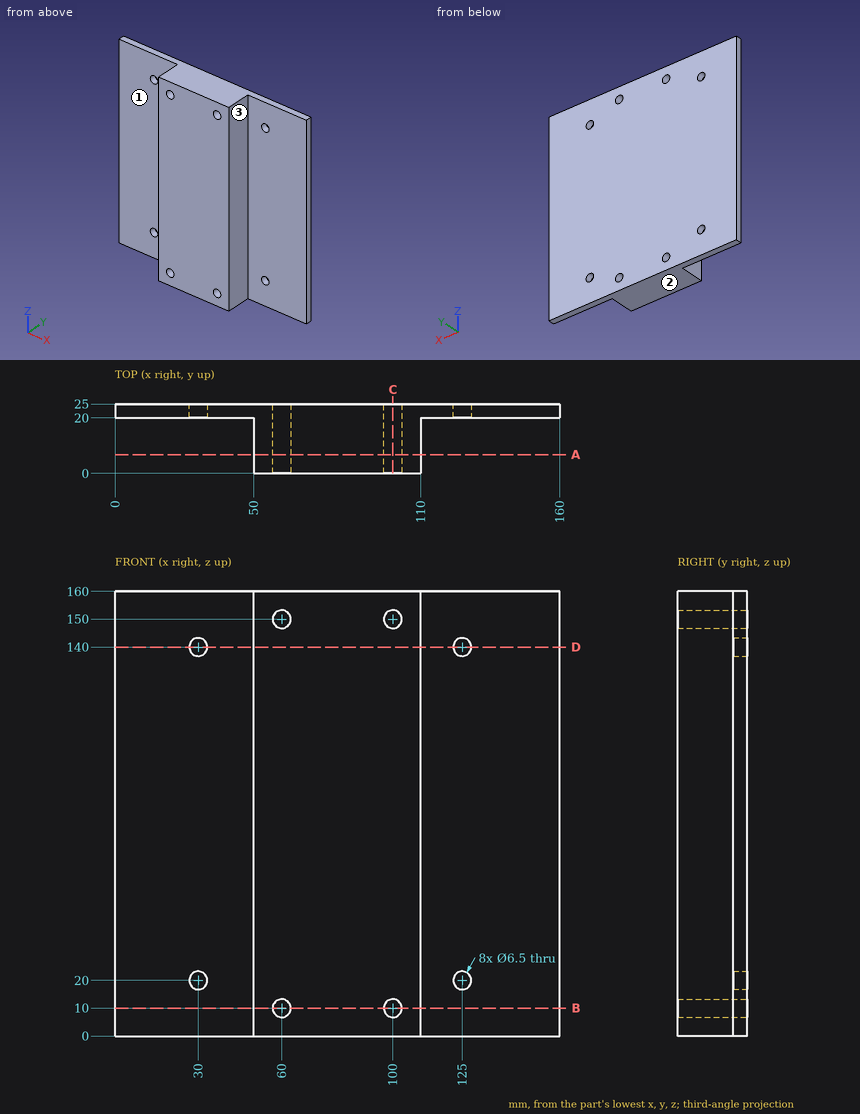
Job drawing, mm, ordinate dimensions from the low corner. One solid piece. A direction names the side the tool comes from. Coordinates: 2 decimals unless noted, no trailing zeros. Order: outer loops, then holes, each group sorted by start corner. A loop starts at its lowest first (then second) coordinate and runs counter-clockwise, first axis right, second up. Notation, with made-up numbers: (-38, 83.25) -> (-32, 83.25) arc R20 ccw to (-32, 118.25) -> close; hole circle Ø11 at (17, 36.5). An arc over 180 degrees is marked (long way). Put each result on its own line as item: value. Start each with the question number.
(1) Band-saw the part on A-A (y = 6.75). Give the cut face in (x, z), then the cut area to 3 significant figures.
(2) Band-saw the part on C-C (x = 100). Give the cut face in (y, z), then the cut area to 4 significant figures.
(3) Band-saw the part on B-B (z = 10). Give the cut face in (x, y), then the cut area to 4 significant figures.
(4) Probe line 1 along Z through (x, y) = (30, 22.05); line 2 along X through (y, z) = (5.5, 150); line 3 along Z through (x, y) = (100, 10). List the from-to ranges inside material, lowest first. Write a range as [from, to].
(5) Which spindle directions (+Z, -Z, +X, -X, +Y, -Y) get a long thin tool onto all of the face, cutting with end or side? Do the marked faces 1, 2 and 3. Say none if no direction does.
(6) Pin check, flat tips, straight feed: pin 1 Ø6 at (y, z) = (8.5, 112.5) entering from -X; pin 2 Ø15 at (x, z) = (135, 95) entering from -Y; pin 3 Ø4 at (x, z) = (30, 140) entering from +Y; pin 4 Ø4 at (y, z) = (15, 133) entering from +X. Stop position of each tip, or through.
(7) Band-saw the part on D-D (z = 140). Give the cut face in (x, y), then the cut area to 4 significant figures.
Determined:
1. outline: (50, 0) -> (110, 0) -> (110, 160) -> (50, 160) -> close; hole circle Ø6.5 at (60, 10); hole circle Ø6.5 at (60, 150); hole circle Ø6.5 at (100, 10); hole circle Ø6.5 at (100, 150)
1. area: 9,470 mm²
2. outline: (0, 0) -> (25, 0) -> (25, 6.75) -> (0, 6.75) -> close; (0, 13.25) -> (25, 13.25) -> (25, 146.75) -> (0, 146.75) -> close; (0, 153.25) -> (25, 153.25) -> (25, 160) -> (0, 160) -> close
2. area: 3,675 mm²
3. outline: (0, 20) -> (50, 20) -> (50, 0) -> (56.75, 0) -> (56.75, 25) -> (0, 25) -> close; (63.25, 0) -> (96.75, 0) -> (96.75, 25) -> (63.25, 25) -> close; (103.25, 0) -> (110, 0) -> (110, 20) -> (160, 20) -> (160, 25) -> (103.25, 25) -> close
3. area: 1,675 mm²
4. line 1: z = [0, 16.75], [23.25, 136.75], [143.25, 160]
4. line 2: x = [50, 56.75], [63.25, 96.75], [103.25, 110]
4. line 3: z = [0, 6.75], [13.25, 146.75], [153.25, 160]
5. face 1: +Z, -Z, -X, -Y
5. face 2: -Z, +X, -X, +Y, -Y
5. face 3: +Z, -Z, +X, -Y
6. pin 1: stops at x = 50
6. pin 2: stops at y = 20
6. pin 3: passes through
6. pin 4: stops at x = 110
7. outline: (0, 20) -> (26.75, 20) -> (26.75, 25) -> (0, 25) -> close; (33.25, 20) -> (50, 20) -> (50, 0) -> (110, 0) -> (110, 20) -> (121.75, 20) -> (121.75, 25) -> (33.25, 25) -> close; (128.25, 20) -> (160, 20) -> (160, 25) -> (128.25, 25) -> close
7. area: 1,935 mm²
